from build123d import *

# Parameters (mm, degrees)
SKETCH1_W           = 50.8
SKETCH1_H           = 25.4
BOSS_EXTRUDE1_DEPTH = 406.4
SHELL1_T            = -3.175
SKETCH2_R           = 14.2875
CUT_EXTRUDE1_DEPTH  = 406.4


with BuildPart() as part:
    # Sketch1 → Boss-Extrude1 (new body)
    with BuildSketch(Plane(origin=(0, 0, 0), x_dir=(1, 0, 0), z_dir=(0, 1, 0))):
        Rectangle(SKETCH1_W, SKETCH1_H)
    extrude(amount=BOSS_EXTRUDE1_DEPTH)

    # Shell1
    shell1_openings = [part.faces().sort_by_distance(p)[0] for p in [
        (0, 406.4, 0),
        (0, 0, 0),
    ]]
    offset(amount=SHELL1_T, openings=shell1_openings, kind=Kind.INTERSECTION)

    # Sketch2 → Cut-Extrude1 (cut)
    with BuildSketch(Plane.XY.offset(12.7)):
        with Locations((0, 387.35)):
            Circle(SKETCH2_R)
    extrude(amount=-CUT_EXTRUDE1_DEPTH, mode=Mode.SUBTRACT)


solid = part.part
Work out the finished part from the listing and answer in its coordinate system (mm). A direction names the side the tool comes from. Coordinates: 2 decimals unless noted, no trailing zeros. Order: outer loops, then holes, each group sorted by start corner. A loop starts at its lowest first (then second) coordinate and runs counter-clockwise, first axis right, second up. Notation, with made-up numbers: (16, 41.25) - (25, 41.25) arc R29 ccw to (25, 79.25) - close; hole circle Ø4 at (26, 27.25). An arc over 180 degrees is marked (long way). Put each result on its own line as item: value. Start each with the question number.
1) Find section D-D (y = 252.5). Give the vertices of the cut face in (x, z) (3 decimals), plus the area to 3 significant figures.
2) For a pull along X with two mould halves and no side action, classify faces 1 (the flat face through (0, 200, -9.525)), 2 (the flat face through (25.4, 200, 0)), 3 (the flat face through (0, 406.4, -10)) as released by +X, released by -X, zero draft, split by the parting line, or undercut.
3) For faces 4 (the flat face through (-22.225, 200, 0)), 5 (the flat face through (0, 200, 12.7)), determine the directions among +Z, -Z, +X, -X, +Y, -Y from which every point of the face is accessible in a straight line to the end or side of a thin tool.
4) Find section C-C (z = -2.25). Give the vertices of the cut face in (x, y) (3 decimals).
5) Find the intervals of material crossed by line 1 (Y direction, x = 0, z = 11.2); line 2 (Z direction, x = 4, y = 226) (3 decimals); line 3 (X direction, y = 202.5, z = -6) (3 decimals), in increasing order. Write a range as from..to.
6) Find section B-B (y = 387.35). Give the vertices of the cut face in (x, z) (1 decimal).
7) Find section A-A (x = 0). Give the vertices of the cut face in (y, z) (1 decimal), plus the area to 3 significant figures.
8) A flat-ended cylindrical pin translates along its axis: pin 1 (12 mm diameter, centred on x = 20, z = 7, fed in from +Y). Find the tip coordinate at first contact, or state that the pin passes through.
Results list:
1. outline: (-25.4, -12.7) - (25.4, -12.7) - (25.4, 12.7) - (-25.4, 12.7) - close; hole (-22.225, -9.525) - (22.225, -9.525) - (22.225, 9.525) - (-22.225, 9.525) - close
1. area: 444 mm^2
2. face 1: undercut
2. face 2: released by +X
2. face 3: zero draft
3. face 4: +Y, -Y
3. face 5: +Z, +X, -X, +Y, -Y
4. outline: (-25.4, 0) - (-22.225, 0) - (-22.225, 406.4) - (-25.4, 406.4) - close; (22.225, 0) - (25.4, 0) - (25.4, 406.4) - (22.225, 406.4) - close
5. line 1: y = 0..373.06, 401.64..406.4
5. line 2: z = -12.7..-9.525, 9.525..12.7
5. line 3: x = -25.4..-22.225, 22.225..25.4
6. outline: (-25.4, -12.7) - (-14.3, -12.7) - (-14.3, -9.5) - (-22.2, -9.5) - (-22.2, 9.5) - (-14.3, 9.5) - (-14.3, 12.7) - (-25.4, 12.7) - close; (14.3, -12.7) - (25.4, -12.7) - (25.4, 12.7) - (14.3, 12.7) - (14.3, 9.5) - (22.2, 9.5) - (22.2, -9.5) - (14.3, -9.5) - close
7. outline: (0, -12.7) - (373.1, -12.7) - (373.1, -9.5) - (0, -9.5) - close; (0, 9.5) - (373.1, 9.5) - (373.1, 12.7) - (0, 12.7) - close; (401.6, -12.7) - (406.4, -12.7) - (406.4, -9.5) - (401.6, -9.5) - close; (401.6, 9.5) - (406.4, 9.5) - (406.4, 12.7) - (401.6, 12.7) - close
7. area: 2,400 mm^2
8. pin 1: stops at y = 406.4
